Geometry check sheet. Reference: the model listing, model coordinates, mm. Face numbers are marked on the shaded views. A direction names the side the tool comes from. Round coordinates to 2 decimals unless told otherwise and drop trailing zeros. Write each loop counter-clockwise with the first axis right and the second up, starting at its lowest first coordinate (ties: lowest second). Pieces come first, ordered by that corner, then holes. Notation, with made-up numbers: (-5, 1) -> (42, 1) arc R14 ccw to (42, 9) -> close; hole circle Ø11 at (-38.75, 26). An arc over 180 degrees is marked (long way). Use a Markdown table: item, result.
```python
from build123d import *

# Parameters (mm, degrees)
BOX001_W               = 32.1
BOX001_H               = 32.1
BOX001_DEPTH           = 114.3
CYLINDER_R             = 4
CYLINDER_DEPTH         = 38.1
CYLINDER_PITCH_ANGLE   = 90
ARRAY001_Z_COUNT       = 3
ARRAY001_Z_PITCH       = 38.1
CYLINDER001_R          = 4
CYLINDER001_DEPTH      = 38.1
CYLINDER001_ROLL_ANGLE = 90
ARRAY_Z_COUNT          = 3
ARRAY_Z_PITCH          = 38.1
BOX_W                  = 38.1
BOX_H                  = 38.1
BOX_DEPTH              = 114.3
FILLET_R               = 1


with BuildPart() as cutout:
    # Box001 → Box001 (new body)
    with BuildSketch(Plane(origin=(3, 3, 0), x_dir=(1, 0, 0), z_dir=(0, 0, 1))):
        with Locations((16.05, 16.05)):
            Rectangle(BOX001_W, BOX001_H)
    extrude(amount=BOX001_DEPTH)


with BuildPart() as holes2:
    # Cylinder → Cylinder (new body)
    with BuildSketch(Plane.XY):
        Circle(CYLINDER_R)
    extrude(amount=CYLINDER_DEPTH)


with BuildPart() as holes2_1:
    # Cylinder pitch: moved
    add(holes2.part.rotate(Axis((0, 0, 0), (0, 1, 0)), CYLINDER_PITCH_ANGLE))


with BuildPart() as holes2_2:
    # Cylinder placement: moved
    add(holes2_1.part.moved(Location((0, 19.05, 19.05))))

    # Array001 Z: Holes2 ×3


with BuildPart() as holes2_3:
    add(holes2_2.part)
    with Locations(*[(0, 0, i * ARRAY001_Z_PITCH) for i in range(1, ARRAY001_Z_COUNT)]):
        add(holes2_2.part)


with BuildPart() as holes1:
    # Cylinder001 → Cylinder001 (new body)
    with BuildSketch(Plane.XY):
        Circle(CYLINDER001_R)
    extrude(amount=CYLINDER001_DEPTH)


with BuildPart() as holes1_1:
    # Cylinder001 roll: moved
    add(holes1.part.rotate(Axis((0, 0, 0), (1, 0, 0)), CYLINDER001_ROLL_ANGLE))


with BuildPart() as holes1_2:
    # Cylinder001 placement: moved
    add(holes1_1.part.moved(Location((19.05, 38.1, 19.05))))

    # Array Z: Holes1 ×3


with BuildPart() as holes1_3:
    add(holes1_2.part)
    with Locations(*[(0, 0, i * ARRAY_Z_PITCH) for i in range(1, ARRAY_Z_COUNT)]):
        add(holes1_2.part)


with BuildPart() as cut002:
    # Box → Box (new body)
    with BuildSketch(Plane.XY):
        with Locations((19.05, 19.05)):
            Rectangle(BOX_W, BOX_H)
    extrude(amount=BOX_DEPTH)

    # Fillet
    fillet_edges = [cut002.edges().sort_by_distance(p)[0] for p in [
        (0, 0, 57.15),
        (38.1, 0, 57.15),
        (38.1, 38.1, 57.15),
        (0, 38.1, 57.15),
    ]]
    fillet(fillet_edges, radius=FILLET_R)

    # Cut: cut Holes1
    add(holes1_3.part, mode=Mode.SUBTRACT)

    # Cut001: cut Holes2
    add(holes2_3.part, mode=Mode.SUBTRACT)

    # Cut002: cut Cutout
    add(cutout.part, mode=Mode.SUBTRACT)


solid = cut002.part
```
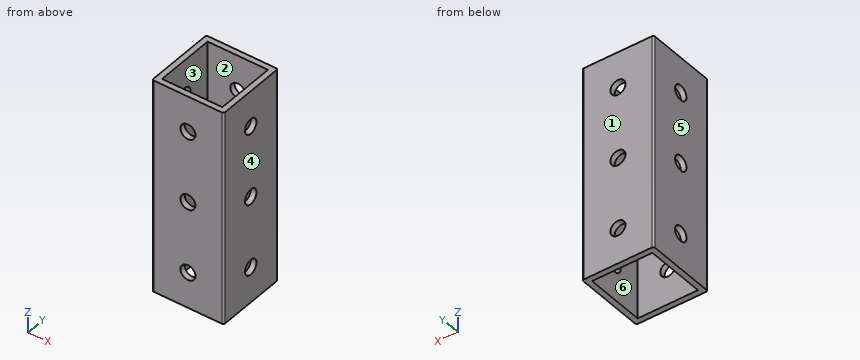
(1) Release check for a two-part mould opening along X. For the marked faces 3, 4, 5 and 6 record: +X half, -X half, draft (parallel to the pull), parting line (faces both ways), or undercut.
A:
| item | result |
|---|---|
| face 3 | undercut |
| face 4 | +X half |
| face 5 | -X half |
| face 6 | undercut |
(2) Section check D-D on x = 19.05. State how many separate pieces and enclosed holes the cut face has, plus the area to 3 significant figures.
A:
| item | result |
|---|---|
| separate pieces | 8 |
| enclosed holes | 0 |
| area | 542 mm2 |
(3) Gauge pin test, flat end, axial feed: pin 1 Ø6.5 at (y, z) = (19.05, 19.05) entering from +X. Record the tip position at first contact, or that the pin passes through.
A:
| item | result |
|---|---|
| pin 1 | passes through |
(4) Access from +Z, -Z, +X, -X, +Y, -Y to the whole of each face (thin tool, end or side, straight path). Record for the marked faces 1 and 2.
A:
| item | result |
|---|---|
| face 1 | +Z, -Z, +X, -X, +Y |
| face 2 | +Z, -Z |
(5) Section check A-A on x = 30.5. Record the cut outline in (y, z), plus the area to 3 significant figures.
A:
| item | result |
|---|---|
| outline | (0, 0) -> (3, 0) -> (3, 114.3) -> (0, 114.3) -> close; (35.1, 0) -> (38.1, 0) -> (38.1, 114.3) -> (35.1, 114.3) -> close |
| area | 686 mm2 |
(6) Thickness scan on line 1 (Z direction, x = 19.05, y = 1.05); line 2 (X direction, y = 22, z = 13). Record the ranges inside material, lowest first.
A:
| item | result |
|---|---|
| line 1 | z = 0 to 15.05, 23.05 to 53.15, 61.15 to 91.25, 99.25 to 114.3 |
| line 2 | x = 0 to 3, 35.1 to 38.1 |
(7) Section check C-C on z = 57.15. Record the cut outline in (x, y).
A:
| item | result |
|---|---|
| outline | (0, 1) arc R1 ccw to (1, 0) -> (15.05, 0) -> (15.05, 3) -> (3, 3) -> (3, 15.05) -> (0, 15.05) -> close; (0, 23.05) -> (3, 23.05) -> (3, 35.1) -> (15.05, 35.1) -> (15.05, 38.1) -> (1, 38.1) arc R1 ccw to (0, 37.1) -> close; (23.05, 0) -> (37.1, 0) arc R1 ccw to (38.1, 1) -> (38.1, 15.05) -> (35.1, 15.05) -> (35.1, 3) -> (23.05, 3) -> close; (23.05, 35.1) -> (35.1, 35.1) -> (35.1, 23.05) -> (38.1, 23.05) -> (38.1, 37.1) arc R1 ccw to (37.1, 38.1) -> (23.05, 38.1) -> close |
